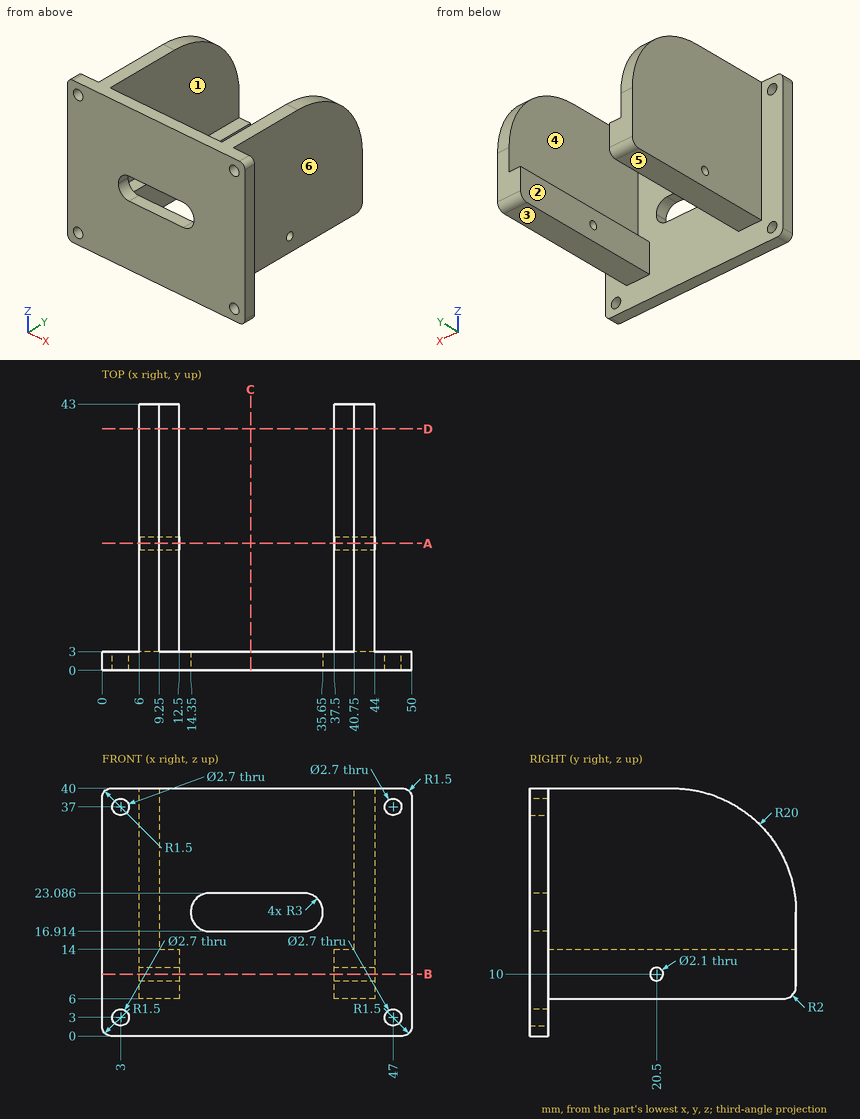
Geometry check sheet. Reference: drawing and pictorial views, mm from the part's lowest x, y, z. A direction names the side the tool comes from. Give positions to 0.01 mm unless a question says otherwise; leave off trailing zeros. Loops run counter-clockwise (first coordinate to the right, second up) from the corner with the lowest first, then second, coordinate; pieces in that order, holes last. Notation, with made-up numbers: M 56,49 L 71,49 A29 cw 71,77 Z; hole C 56,-29.5 d4. An arc over 180 degrees is marked long. Use a Markdown table: item, result. Add a question column.
Q1. Sectioned sample at D-D, the plane y = 39. Record the cut outline in (x, z), then the cut area to 3 significant figures.
Q2. Sectioned sample at C-C, the plane x = 24. Record the cut outline in (y, z).
Q3. Mould release check, pull along X, two halves, no side actions. Record for the marked faces 4, 5 and 6: pulls with the +X half, pulls with the -X half, needs draft (parallel to the pull), parting line crosses it, or undercut.
Q4. Sectioned sample at B-B, the plane z = 10. Record the cut outline in (x, y), then the cut area to 3 significant figures.
Q5. Tool access check on the marked faces 1, 2 and 3. Record the directions out of +Z, -Z, +X, -X, +Y, -Y that give a thin tool (end or side, any length) a straight path to the whole face; none if there is none.
Q6. Go/stop test with flat-tipped pins: pin 1 (3 mm diameter, centred on x = 47, z = 3, fed in from +Y); pin 2 (2.5 mm diameter, centred on y = 20.5, z = 10, fed in from -X); pin 3 (9 mm diameter, centred on y = 30.5, z = 11.5, fed in from +X). Record where each tip stops, or that it passes through.
Q7. Sectioned sample at A-A, the plane y = 20.5. Record the cut outline in (x, z).
Q8. Scan lines: line 1 along X through (y, z) = (24.5, 34); line 2 along X through (y, z) = (0.7, 3); line 3 along X through (y, z) = (14.5, 8). Record each from-to range of solid material in increasing order. Write a range as [from, to].
Verdict:
| question | item | result |
|---|---|---|
| 1 | outline | M 6,6 L 12.5,6 L 12.5,14 L 9.25,14 L 9.25,32 L 6,32 Z; M 37.5,6 L 44,6 L 44,32 L 40.75,32 L 40.75,14 L 37.5,14 Z |
| 1 | area | 221 mm^2 |
| 2 | outline | M 0,0 L 3,0 L 3,16.91 L 0,16.91 Z; M 0,23.09 L 3,23.09 L 3,40 L 0,40 Z |
| 3 | face 4 | undercut |
| 3 | face 5 | needs draft |
| 3 | face 6 | pulls with the +X half |
| 4 | outline | M 0,0 L 50,0 L 50,3 L 44,3 L 44,19.45 L 37.5,19.45 L 37.5,3 L 12.5,3 L 12.5,19.45 L 6,19.45 L 6,3 L 0,3 Z; M 6,21.55 L 12.5,21.55 L 12.5,43 L 6,43 Z; M 37.5,21.55 L 44,21.55 L 44,43 L 37.5,43 Z |
| 4 | area | 643 mm^2 |
| 5 | face 1 | +Z, +Y |
| 5 | face 2 | +Z, -Z, +Y |
| 5 | face 3 | -Z, +X, -X, +Y |
| 6 | pin 1 | y = 3 |
| 6 | pin 2 | x = 6 |
| 6 | pin 3 | x = 44 |
| 7 | outline | M 6,6 L 12.5,6 L 12.5,8.95 L 6,8.95 Z; M 6,11.05 L 12.5,11.05 L 12.5,14 L 9.25,14 L 9.25,40 L 6,40 Z; M 37.5,6 L 44,6 L 44,8.95 L 37.5,8.95 Z; M 37.5,11.05 L 44,11.05 L 44,40 L 40.75,40 L 40.75,14 L 37.5,14 Z |
| 8 | line 1 | [6, 9.25], [40.75, 44] |
| 8 | line 2 | [0, 1.65], [4.35, 45.65], [48.35, 50] |
| 8 | line 3 | [6, 12.5], [37.5, 44] |
